CAD build for the part. Positions are in the model's coordinates, mm. Give positions to 0.01 mm unless a question says otherwise; leave off trailing zeros. Loops run counter-clockwise (first coordinate to the right, second up) from the corner with the lowest first, then second, coordinate; pieces in that order, holes last.
Item 1: Saw through at B-B on x = 0. Give the cut face in (y, z), plus the area to 3 significant figures.
Item 2: Probe probe 1 along Y at (x, z) = (-7, 0.75); probe 2 along X at (y, z) = (-5.5, 0.55); probe 3 along X at (y, z) = (-7.5, 0.35). List the from-to ranges inside material, lowest first.
Item 3: Saw through at D-D on x = -27. Give the cut face in (y, z).
Item 4: Saw through at A-A on z = 3.4. Give the cut face in (x, y), plus the area to 3 significant figures.
Item 5: Saw through at C-C on y = 34.7. Give the cut face in (x, z), plus the area to 3 significant figures.
Item 6: Drop flat-ended pins along their axis: P1, Ø2.5, axis at x = 33.5, z = 3.5, coming from the -Y side; P2, Ø0.9, axis at y = -24.5, z = 3, coming from the +X side; P3, Ø0.9, axis at x = -33, z = 2.5, coming from the +Y side. Give the stop position or say it passes through.
from build123d import *

# Parameters (mm, degrees)
PAD_DEPTH             = 1.2
POCKET_DEPTH          = 208.145687
POLARPATTERN_COUNT    = 4
POCKET001_DEPTH       = 1.201
SKETCH003_W           = 3
SKETCH003_H           = 3
PAD001_DEPTH          = 3
POLARPATTERN001_COUNT = 2


with BuildPart() as part:
    # Sketch → Pad (new body)
    with BuildSketch(Plane.XY):
        with BuildLine():
            Line((36.5, 27), (36.5, -27))
            Line((36.5, -27), (-36.5, -27))
            Line((-36.5, -27), (-36.5, 27))
            Line((-36.5, 27), (-5.660898, 44.804964))
            ThreePointArc((5.660898, 44.804964), (0, 46.321797), (-5.660898, 44.804964))
            Line((5.660898, 44.804964), (36.5, 27))
        make_face()
    extrude(amount=PAD_DEPTH)

    # Sketch001 (on Face8 of Pad) → Pocket (cut, through all)
    with BuildSketch(Plane.XY.offset(1.2)):
        with BuildLine():
            Line((-24, 17.5), (-24, -17.5))
            Line((-13.093649, -9.863291), (-24, -17.5))
            ThreePointArc((-13.093649, -9.863291), (-7.959145, 0), (-13.093649, 9.863291))
            Line((-13.093649, 9.863291), (-24, 17.5))
        make_face()
    pocket = extrude(amount=-POCKET_DEPTH, mode=Mode.SUBTRACT)

    # PolarPattern: Pocket ×4 about axis
    polarpattern_axis = Axis((0, 0, 1.2), (0, 0, 1))
    for i in range(1, POLARPATTERN_COUNT):
        add(pocket.rotate(polarpattern_axis, i * 360 / POLARPATTERN_COUNT), mode=Mode.SUBTRACT)

    # Sketch002 (on Face5 of PolarPattern) → Pocket001 (cut, through all)
    with BuildSketch(Plane.XY.offset(1.2)):
        with BuildLine():
            Line((-2.2, 38.625557), (-2.2, 41.399983))
            ThreePointArc((2.2, 41.399982), (1e-06, 43.6), (-2.2, 41.399983))
            Line((2.2, 38.625557), (2.2, 41.399982))
            ThreePointArc((-2.2, 38.625557), (0, 30.2), (2.2, 38.625557))
        make_face()
    extrude(amount=-POCKET001_DEPTH, mode=Mode.SUBTRACT)

    # Sketch003 (on Face5 of Pocket001) → Pad001 (join)
    with BuildSketch(Plane.XY.offset(1.2)):
        with Locations((-33.8, -24.3)):
            Rectangle(SKETCH003_W, SKETCH003_H)
    pad001 = extrude(amount=PAD001_DEPTH)

    # PolarPattern001: Pad001 ×2 about axis
    polarpattern001_axis = Axis((0, 0, 1.2), (0, 0, 1))
    for i in range(1, POLARPATTERN001_COUNT):
        add(pad001.rotate(polarpattern001_axis, i * 360 / POLARPATTERN001_COUNT))

    # Mirrored: Pad001 across YZ
    add(pad001.mirror(Plane.YZ))

    # Mirrored001: Pad001 across XZ
    add(pad001.mirror(Plane.XZ))


solid = part.part
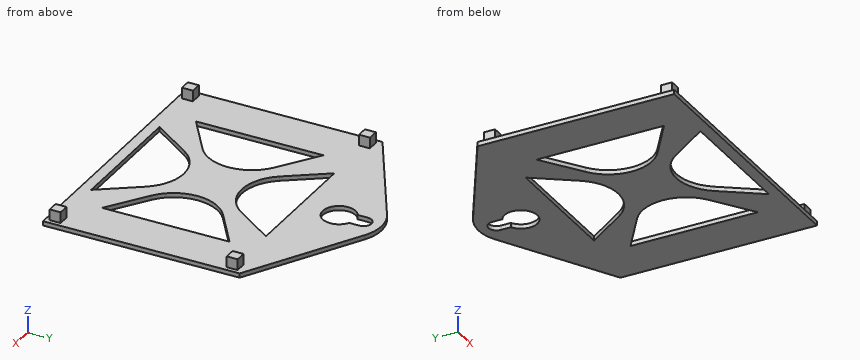
Results below:
1. outline: (-27, 0) - (-24, 0) - (-24, 1.2) - (-27, 1.2) - close; (-7.96, 0) - (7.96, 0) - (7.96, 1.2) - (-7.96, 1.2) - close; (24, 0) - (30.2, 0) - (30.2, 1.2) - (24, 1.2) - close; (43.6, 0) - (46.32, 0) - (46.32, 1.2) - (43.6, 1.2) - close
1. area: 33.4 mm2
2. probe 1: y = -27 to -24, -10.2 to 10.2, 24 to 44.03
2. probe 2: x = -36.5 to -24, -9.29 to 9.29, 24 to 36.5
2. probe 3: x = -36.5 to -24, -10.58 to 10.58, 24 to 36.5
3. outline: (-27, 0) - (32.48, 0) - (32.48, 1.2) - (-27, 1.2) - close
4. outline: (-35.3, -25.8) - (-32.3, -25.8) - (-32.3, -22.8) - (-35.3, -22.8) - close; (-35.3, 22.8) - (-32.3, 22.8) - (-32.3, 25.8) - (-35.3, 25.8) - close; (32.3, -25.8) - (35.3, -25.8) - (35.3, -22.8) - (32.3, -22.8) - close; (32.3, 22.8) - (35.3, 22.8) - (35.3, 25.8) - (32.3, 25.8) - close
4. area: 36.0 mm2
5. outline: (-23.16, 0) - (-4.5, 0) - (-4.5, 1.2) - (-23.16, 1.2) - close; (4.5, 0) - (23.16, 0) - (23.16, 1.2) - (4.5, 1.2) - close
5. area: 44.8 mm2
6. P1: stops at y = -25.8
6. P2: stops at x = 35.3
6. P3: stops at y = 25.8
